Input: part model. Units: mm. Frame: model coordinates. Coordinates: 2 decimals unless noted, no trailing zeros. Use a Markdown table: item, result. Add a question column.
Q1. Material intervals for probe 1 along Z at (x, y) = (-0.5, 4.75); probe 2 along X at (y, z) = (-9, 3), sorted ascending. Write a range as from..to.
Q2. Pin query (flat end, axial travel): P1, Ø12, axis at y = 8.5, z = 0, coming from the -X side; P2, Ø1.5, axis at y = -4, z = 5, coming from the -X side; P3, Ø1.5, axis at x = 5.5, z = 9, coming from the +Y side; P4, Ø13, axis at x = 0, z = 0, coming from the -Y side. Return the tip coordinate at first contact, or that it passes through.
Q3. Mould query, pull axis X, two halves, no side actions, for faces 1 (the face through (0, 0, 11.43)), 2 (the face through (-5.037, -0.163, 0.661)). Classes: released by +X, released by -X, zero draft, split by the parting line, or undercut.
from build123d import *
from build123d.topology import SkipClean

# Parameters (mm, degrees)
SKETCH1_R               = 12.7
BOSS_EXTRUDE1_DEPTH     = 12.7
FILLET1_R               = 12.7
BOSS_EXTRUDE2_START     = 12.7
SKETCH2_R               = 12.7
BOSS_EXTRUDE2_DEPTH     = 12.7
FILLET2_R               = 12.7
CUT_EXTRUDE1_DEPTH      = 22.997045372
CUT_EXTRUDE1_DEPTH_BACK = 22.997045372
SKETCH3_R               = 5.08
CUT_EXTRUDE2_DEPTH      = 22.402439379
CUT_EXTRUDE2_DEPTH_BACK = 22.402439379
SKETCH5_W               = 27.579814606
SKETCH5_H               = 6.012661004


with BuildPart() as part:
    # Sketch1 → Boss-Extrude1 (new body)
    with BuildSketch(Plane(origin=(0, 0, 0), x_dir=(1, 0, 0), z_dir=(0, 1, 0))):
        with Locations(Location((0, 0, 0), (0, 0, 270))):
            Circle(SKETCH1_R)
    extrude(amount=BOSS_EXTRUDE1_DEPTH)

    # Fillet1
    fillet1_edges = [part.edges().sort_by_distance(p)[0] for p in [
        (0, 12.7, -12.7),
    ]]
    fillet(fillet1_edges, radius=FILLET1_R - 0.0001)  # a hair under: the kernel refuses the full size

    # Sketch2 → Boss-Extrude2 (add)
    with SkipClean():  # the faces are left unmerged after this step: merging them gives an invalid solid
        with BuildSketch(Plane.XZ.offset(BOSS_EXTRUDE2_START)):
            with Locations(Location((0, 0, 0), (0, 0, 270))):
                Circle(SKETCH2_R)
        extrude(amount=-BOSS_EXTRUDE2_DEPTH)

    # Fillet2
    fillet2_edges = [part.edges().sort_by_distance(p)[0] for p in [
        (0, -12.7, 12.7),
    ]]
    fillet(fillet2_edges, radius=FILLET2_R - 0.0001)  # a hair under: the kernel refuses the full size

    # Sketch3 → Cut-Extrude1 (cut, two sides: drawn at the far end of the back side and taken through both)
    with BuildSketch(Plane(origin=(0, 0, 0), x_dir=(1, 0, 0), z_dir=(0, 1, 0)).offset(-CUT_EXTRUDE1_DEPTH_BACK)):
        with Locations(Location((0, 0, 0), (0, 0, 90))):
            Circle(SKETCH3_R)
    extrude(amount=CUT_EXTRUDE1_DEPTH + CUT_EXTRUDE1_DEPTH_BACK, mode=Mode.SUBTRACT)

    # Sketch5 → Cut-Extrude2 (cut, two sides: drawn at the far end of the back side and taken through both)
    with BuildSketch(Plane(origin=(0, 0, 0), x_dir=(1, 0, 0), z_dir=(0, 1, 0)).offset(-CUT_EXTRUDE2_DEPTH_BACK)):
        with Locations((0.71890512, -14.436330502)):
            Rectangle(SKETCH5_W, SKETCH5_H)
    extrude(amount=CUT_EXTRUDE2_DEPTH + CUT_EXTRUDE2_DEPTH_BACK, mode=Mode.SUBTRACT)


solid = part.part
Values follow:
| question | item | result |
|---|---|---|
| 1 | probe 1 | -11.77..-5.06, 5.06..11.43 |
| 1 | probe 2 | -8.44..-4.1, 4.1..8.44 |
| 2 | P1 | x = -12.45 |
| 2 | P2 | x = -11.37 |
| 2 | P3 | y = 8.08 |
| 2 | P4 | y = -11.64 |
| 3 | face 1 | zero draft |
| 3 | face 2 | undercut |
